```python
from build123d import *

# Parameters (mm, degrees)
F1_DEPTH = 50
F2_W     = 11
F2_H     = 10
F3_DEPTH = 2
F4_W     = 11
F4_H     = 10
F5_DEPTH = 2


with BuildPart() as f1:
    # F0 (on Front) → F1 (new body)
    with BuildSketch(Plane.XZ):
        with BuildLine():
            Line((0, 10), (0, 0))
            Line((0, 0), (2, 0))
            Line((2, 0), (2, 5.5))
            ThreePointArc((2, 5.5), (5.5, 9), (9, 5.5))
            Line((9, 5.5), (9, 0))
            Line((9, 0), (11, 0))
            Line((11, 0), (11, 10))
            Line((11, 10), (0, 10))
        make_face()
    extrude(amount=F1_DEPTH)

    # F2 (on face) → F3 (join)
    with BuildSketch(Plane(origin=(0, 0, 0), x_dir=(-1, 0, 0), z_dir=(0, 1, 0))):
        with Locations((-5.5, 5)):
            Rectangle(F2_W, F2_H)
    extrude(amount=F3_DEPTH)

    # F4 (on face) → F5 (join)
    with BuildSketch(Plane.XZ.offset(50)):
        with Locations((5.5, 5)):
            Rectangle(F4_W, F4_H)
    extrude(amount=F5_DEPTH)


solid = f1.part
```
Check sheet for the modelled part. Datum: model origin and axes. Units: mm. A direction names the side the tool comes from. Give positions to 0.01 mm unless a question says otherwise; leave off trailing zeros. Write each loop counter-clockwise with the first axis right and the second up, starting at its lowest first coordinate (ties: lowest second). Pieces come first, ordered by that corner, then holes.
Item 1: Cross-section at C-C (y = -28.5). Enter the section's corners in (x, z).
Item 2: Scan lines: L1, parallel to X at y = -28.5, z = 3.75; L2, parallel to Y at x = 4.25, z = 4.75; L3, parallel to X at y = -32.5, z = 7.75. Record each from-to range of solid material in increasing order.
Item 3: Gauge pin test, flat ends, axial feed: pin 1 (3 mm diameter, centred on x = 7, y = -15, fed in from -Z); pin 2 (1.5 mm diameter, centred on y = -26, z = 8, fed in from -X). Record the tip position at first contact, or that the pin passes through.
Item 4: Cross-section at A-A (z = 1.5). Enter the section's corners in (x, y).
Item 5: Draft check along X on faces 3 (the face through (6, 2, 5)), 4 (the face through (5, -50, 5)), 5 (the face through (2, -25, 3)), 6 (the face through (11, -25, 5)). Enter one of: released by +X, released by -X, zero draft, split by the parting line, or undercut.
Item 6: Cross-section at B-B (x = 5.5). Enter the section's corners in (y, z), and give its area (3 significant figures).
Item 7: Cross-section at D-D (z = 6.5). Enter the section's corners in (x, y).
Item 8: Access from +Z, -Z, +X, -X, +Y, -Y to the whole of each face (thin tool, end or side, straight path). Record for faces 1 (the face through (5, -25, 10)), 2 (the face through (5.4, -24.6, 9)).
Report:
1. outline: (0, 0) - (2, 0) - (2, 5.5) arc R3.5 cw to (9, 5.5) - (9, 0) - (11, 0) - (11, 10) - (0, 10) - close
2. L1: x = 0 to 2, 9 to 11
2. L2: y = -52 to -50, 0 to 2
2. L3: x = 0 to 2.82, 8.18 to 11
3. pin 1: stops at z = 7.3
3. pin 2: stops at x = 0
4. outline: (0, -52) - (11, -52) - (11, 2) - (0, 2) - close; hole (2, -50) - (9, -50) - (9, 0) - (2, 0) - close
5. face 3: zero draft
5. face 4: undercut
5. face 5: undercut
5. face 6: released by +X
6. outline: (-52, 0) - (-50, 0) - (-50, 9) - (0, 9) - (0, 0) - (2, 0) - (2, 10) - (-52, 10) - close
6. area: 90.0 mm2
7. outline: (0, -52) - (11, -52) - (11, 2) - (0, 2) - close; hole (2.15, -50) - (8.85, -50) - (8.85, 0) - (2.15, 0) - close
8. face 1: +Z, +X, -X, +Y, -Y
8. face 2: -Z
